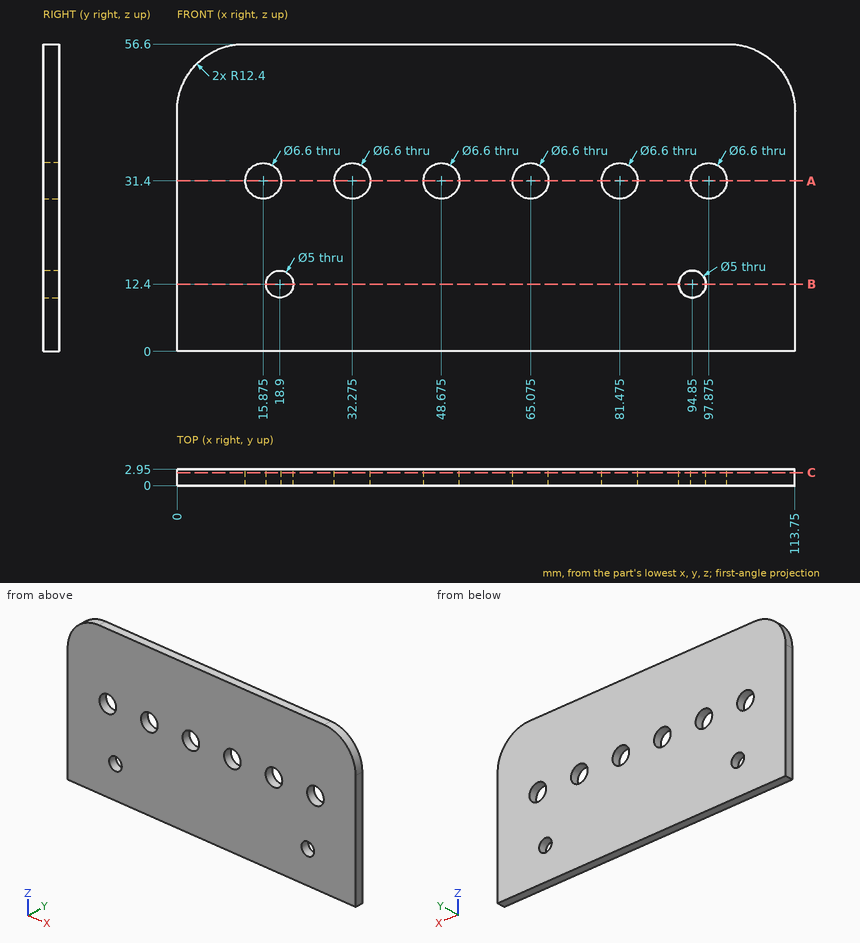
For this review, use the dimensioned drawing (mm, ordinates from the lowest corner) and the shaded views. Coordinates: 2 decimals unless noted, no trailing zeros. Order: outer loops, then holes, each group sorted by start corner. A loop starts at its lowest first (then second) coordinate and runs counter-clockwise, first axis right, second up. Notation, with made-up numbers: M 71.25,34.25 L 107.25,34.25 A21 cw 107.25,51.25 Z; hole C -30,-17.75 d8. An arc over 180 degrees is marked long. Answer as a JSON object with one key per item and string values. Group by question number.
1) Add section A-A, the plane z = 31.4. Write out the cut boundary in (x, y) (3 decimals).
2) Wall thickness on L1, parallel to X at y = 1.7, z = 12.5; L2, parallel to X at y = 2.6, z = 13; L3, parallel to Z at x = 17.5, y = 1.75: over which ranges is each line inside the solid? List them lowest first.
3) For pin 1 (1.5 mm diameter, centred on y = 1, z = 47.5, fed in from +X) (3 decimals), flat-tipped, find the tip position at first contact; note if it passes through.
4) Add section B-B, the plane z = 12.4. Write out the cut boundary in (x, y).
5) Add section C-C, the plane y = 2.35. Count the separate pieces of the cut face and the enclosed holes in it, then the cut area to 3 significant figures.
Computed values:
{
 "1": {"outline": "M 0,0 L 12.575,0 L 12.575,2.95 L 0,2.95 Z; M 19.175,0 L 28.975,0 L 28.975,2.95 L 19.175,2.95 Z; M 35.575,0 L 45.375,0 L 45.375,2.95 L 35.575,2.95 Z; M 51.975,0 L 61.775,0 L 61.775,2.95 L 51.975,2.95 Z; M 68.375,0 L 78.175,0 L 78.175,2.95 L 68.375,2.95 Z; M 84.775,0 L 94.575,0 L 94.575,2.95 L 84.775,2.95 Z; M 101.175,0 L 113.75,0 L 113.75,2.95 L 101.175,2.95 Z"},
 "2": {"L1": "x = 0 to 16.4, 21.4 to 92.35, 97.35 to 113.75", "L2": "x = 0 to 16.47, 21.33 to 92.42, 97.28 to 113.75", "L3": "z = 0 to 10.33, 14.47 to 28.53, 34.27 to 56.6"},
 "3": {"pin 1": "stops at x = 113.485"},
 "4": {"outline": "M 0,0 L 16.4,0 L 16.4,2.95 L 0,2.95 Z; M 21.4,0 L 92.35,0 L 92.35,2.95 L 21.4,2.95 Z; M 97.35,0 L 113.75,0 L 113.75,2.95 L 97.35,2.95 Z"},
 "5": {"separate pieces": "1", "enclosed holes": "8", "area": "6,130 mm^2"}
}
